Drawing for the job (mm, zero at the part's lowest x, y, z). Round coordinates to 2 decimals unless told otherwise and drop trailing zeros. Loops run counter-clockwise (first coordinate to the right, second up) from the corner with the lowest first, then second, coordinate; pieces in that order, holes last. Notation, with made-up numbers: (-7, 29.25) - (40, 29.25) arc R29 cw to (40, 62.25) - close; hole circle Ø9 at (86, -23.5). An arc over 180 degrees is marked (long way). Put each result on its own line as item: value.
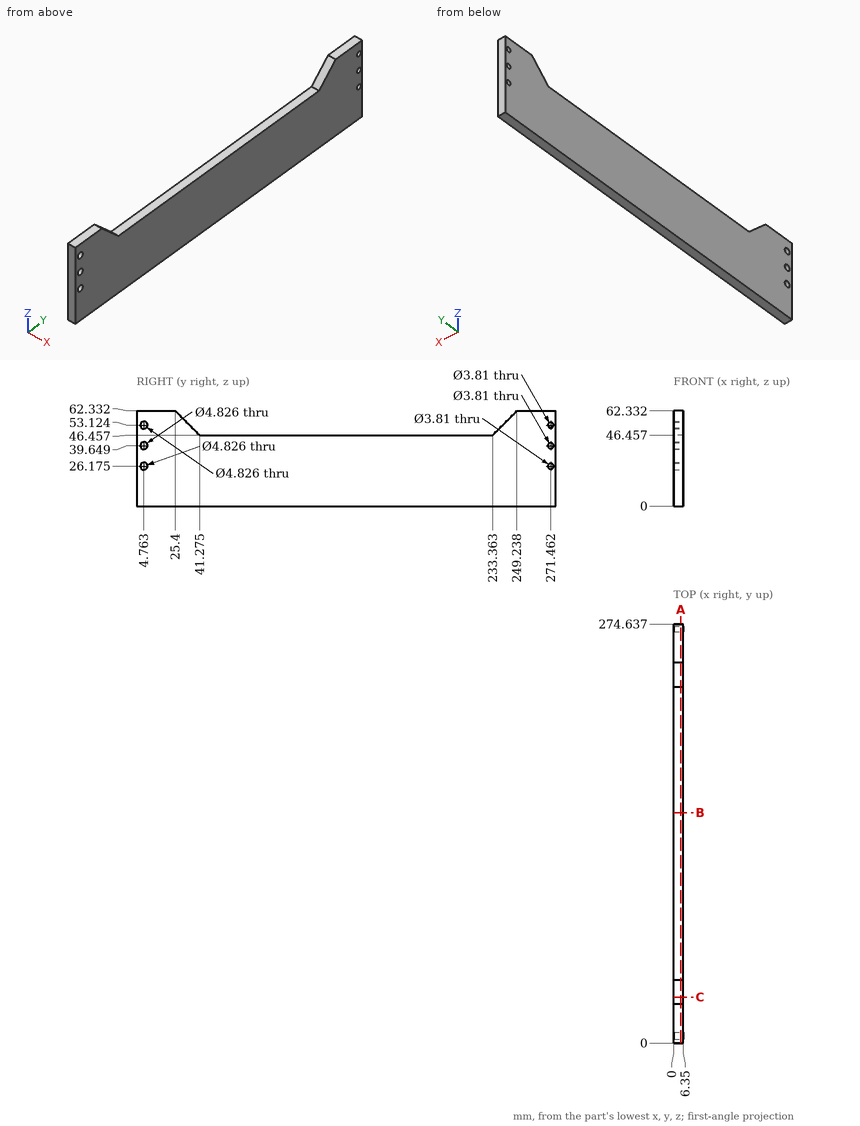
1. Probe line 1 along Y through (x, z) = (4.25, 39.5) (1 decimal); line 2 along Z through (x, y) = (1.25, 159); line 3 along Z through (x, y) = (1.25, 234) (1 decimal). List the from-to ranges inside material, lowest first. Write a range as [from, to].
A:
line 1: y = [0, 2.4], [7.2, 269.6], [273.4, 274.6]
line 2: z = [0, 46.46]
line 3: z = [0, 47.1]
2. Band-saw the part on B-B (y = 151). List the corners of the cut face in (x, z), plus the area to 3 significant figures.
A:
outline: (0, 0) - (6.35, 0) - (6.35, 46.46) - (0, 46.46) - close
area: 295 mm²
3. Band-saw the part on A-A (x = 4.75). Give the number of separate pieces and of enclosed holes in the cut face, plus the area to 3 significant figures.
A:
separate pieces: 1
enclosed holes: 6
area: 13,700 mm²
4. Band-saw the part on C-C (y = 30). List the corners of the cut face in (x, z).
A:
outline: (0, 0) - (6.35, 0) - (6.35, 57.73) - (0, 57.73) - close
